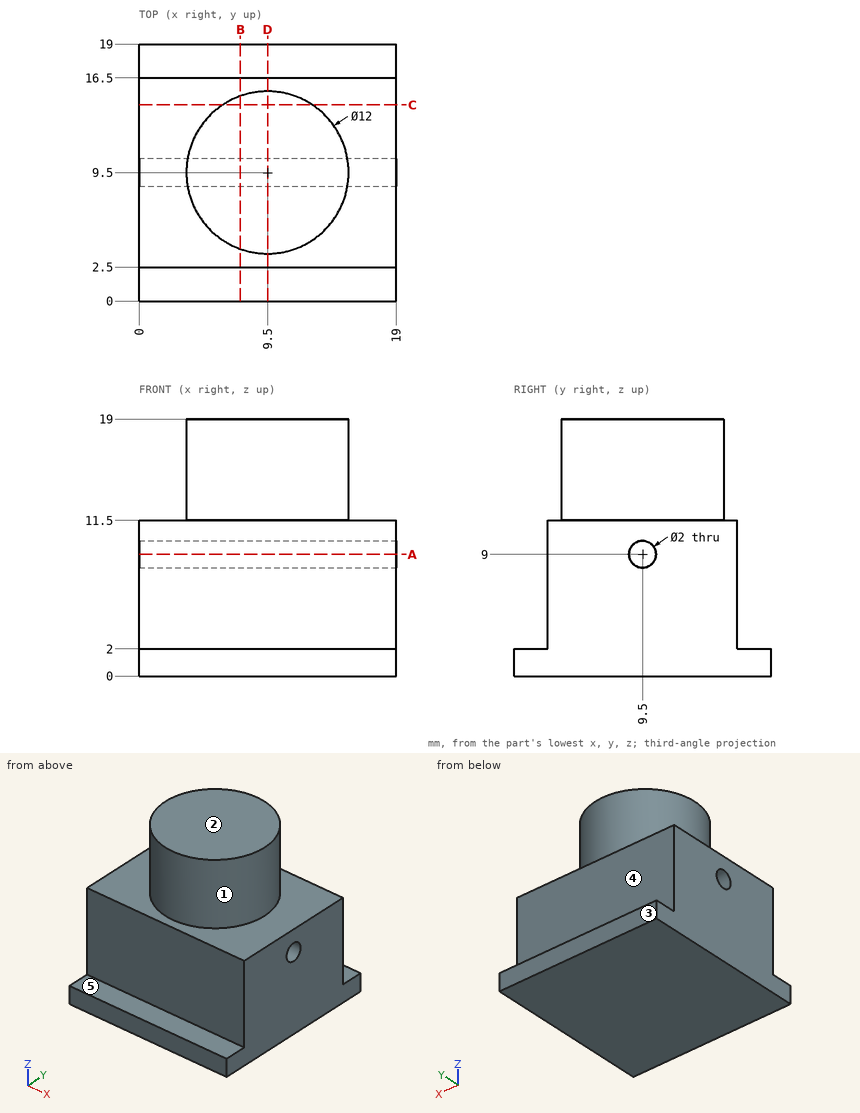
Check sheet for the drawn part. Datum: minimum x, y, z corner. Units: mm. A direction names the side the tool comes from. Round coordinates to 2 decimals unless told otherwise and drop trailing zeros. Loops run counter-clockwise (first coordinate to the right, second up) from the corner with the lowest first, then second, coordinate; pieces in that order, holes last. Notation, with made-up numbers: (75.25, -4) - (109.25, -4) arc R19 cw to (109.25, 26) - close; hole circle Ø4 at (23.25, -4.5). An arc over 180 degrees is marked (long way). Write each question's results on one line, items separated by ' | '. Start each with the question number.
Q1. Thickness scan on line 1 (Y direction, x = 10.75, z = 9); line 2 (Z direction, x = 14.75, y = 9.5); line 3 (Y direction, x = 10.5, z = 4.5). Record the ranges inside material, lowest first. Write a range as [from, to].
Q2. Cross-section at B-B on x = 7.5. Enter the section's corners in (y, z).
Q3. Cross-section at D-D on x = 9.5. Enter the section's corners in (y, z), and give its area (3 significant figures).
Q4. Cross-section at C-C on y = 14.5. Enter the section's corners in (x, z), and give its area (3 significant figures).
Q5. Cross-section at A-A on z = 9. Enter the section's corners in (x, y), and give its area (3 significant figures).
Q6. Access from +Z, -Z, +X, -X, +Y, -Y to the whole of each face (thin tool, end or side, straight path). Record for the marked faces 1, 2, 3, 4 and 5.
Q7. Gauge pin test, flat ends, axial feed: P1, Ø10.5, axis at x = 10, z = 7.5, coming from the +Y side; P2, Ø2, axis at x = 17, y = 9.5, coming from the +Z side; P3, Ø1.8, axis at y = 9.5, z = 9, coming from the -X side; P4, Ø0.8, axis at x = 5, y = 17, coming from the +Z side. Record the tip position at first contact, or that the pin passes through.
Answers below:
1) line 1: y = [2.5, 8.5], [10.5, 16.5] | line 2: z = [0, 8], [10, 19] | line 3: y = [2.5, 16.5]
2) outline: (0, 0) - (19, 0) - (19, 2) - (16.5, 2) - (16.5, 11.5) - (15.16, 11.5) - (15.16, 19) - (3.84, 19) - (3.84, 11.5) - (2.5, 11.5) - (2.5, 2) - (0, 2) - close; hole circle Ø2 at (9.5, 9)
3) outline: (0, 0) - (19, 0) - (19, 2) - (16.5, 2) - (16.5, 11.5) - (15.5, 11.5) - (15.5, 19) - (3.5, 19) - (3.5, 11.5) - (2.5, 11.5) - (2.5, 2) - (0, 2) - close; hole circle Ø2 at (9.5, 9) | area: 258 mm²
4) outline: (0, 0) - (19, 0) - (19, 11.5) - (12.82, 11.5) - (12.82, 19) - (6.18, 19) - (6.18, 11.5) - (0, 11.5) - close | area: 268 mm²
5) outline: (0, 2.5) - (19, 2.5) - (19, 8.5) - (0, 8.5) - close; (0, 10.5) - (19, 10.5) - (19, 16.5) - (0, 16.5) - close | area: 228 mm²
6) face 1: +Z | face 2: +Z, +X, -X, +Y, -Y | face 3: +Z, -Z, +X, -X, +Y | face 4: +Z, +X, -X, +Y | face 5: +Z, +X, -X, -Y
7) P1: stops at y = 16.5 | P2: stops at z = 11.5 | P3: passes through | P4: stops at z = 2
